Model file for the job. Use its own axes, mm. Round coordinates to 2 decimals unless told otherwise and drop trailing zeros. Order: outer loops, then holes, each group sorted by start corner. A loop starts at its lowest first (then second) coordinate and runs counter-clockwise, first axis right, second up. Notation, with made-up numbers: (22.25, 1) - (79.25, 1) arc R19 ccw to (79.25, 14) - close; hole circle Ø9 at (27.25, 5). An arc over 180 degrees is marked (long way). Write item = value, one per line. Start each with the question number.
from build123d import *

# Parameters (mm, degrees)
SKETCH1_W           = 51
SKETCH1_H           = 28
BOSS_EXTRUDE1_DEPTH = 3
SKETCH2_R           = 1.6
CUT_EXTRUDE1_DEPTH  = 3
SKETCH3_R           = 3.1
CUT_EXTRUDE2_DEPTH  = 3


with BuildPart() as part:
    # Sketch1 → Boss-Extrude1 (new body)
    with BuildSketch(Plane(origin=(0, 0, 0), x_dir=(1, 0, 0), z_dir=(0, 1, 0))):
        with Locations((-1.082278481, 0.240506329)):
            Rectangle(SKETCH1_W, SKETCH1_H)
    extrude(amount=BOSS_EXTRUDE1_DEPTH)

    # Sketch2 → Cut-Extrude1 (cut)
    with BuildSketch(Plane(origin=(0, 3, 0), x_dir=(1, 0, 0), z_dir=(0, 1, 0))):
        with Locations((-23.582278481, 11.240506329)):
            Circle(SKETCH2_R)
        with Locations((21.417721519, 11.240506329)):
            Circle(SKETCH2_R)
    extrude(amount=-CUT_EXTRUDE1_DEPTH, mode=Mode.SUBTRACT)

    # Sketch3 → Cut-Extrude2 (cut)
    with BuildSketch(Plane(origin=(0, 3, 0), x_dir=(1, 0, 0), z_dir=(0, 1, 0))):
        with Locations((-1.582278481, 0.240506329)):
            Circle(SKETCH3_R)
    extrude(amount=-CUT_EXTRUDE2_DEPTH, mode=Mode.SUBTRACT)


solid = part.part
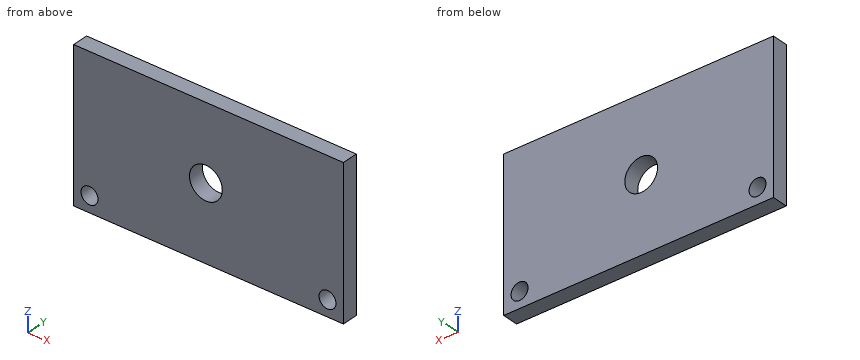
Item 1: Saw through at A-A, the plane z = -2.25. Give the cut face in (x, y).
Item 2: Drop flat-ended pins along their axis: pin 1 (8 mm diameter, centred on x = 4.5, z = 8, fed in from -Y); pin 2 (5.5 mm diameter, centred on x = -1.58, z = -0.24, fed in from -Y). Give the stop position or say it passes through.
Item 3: Probe L1, parallel to X at y = 2.4, z = -12.5; L2, parallel to X at y = 2.4, z = -10.5; L3, parallel to Z at x = 0.5, y = 1.65. List the from-to ranges inside material, lowest first.
Item 4: Saw through at B-B, the plane y = 0.9. Give the cut face in (x, z), then the cut area to 3 significant figures.
Item 5: Saw through at C-C, the plane x = -3.5. Give the cut face in (y, z), then the cut area to 3 significant figures.
Check sheet entries:
q1.outline = (-26.58, 0) - (-3.94, 0) - (-3.94, 3) - (-26.58, 3) - close; (0.78, 0) - (24.42, 0) - (24.42, 3) - (0.78, 3) - close
q2.pin_1 = 0
q2.pin_2 = through
q3.L1 = -26.58 to -24.57, -22.6 to 20.43, 22.4 to 24.42
q3.L2 = -26.58 to -25, -22.16 to 20, 22.84 to 24.42
q3.L3 = -14.24 to -2.54, 2.06 to 13.76
q4.outline = (-26.58, -14.24) - (24.42, -14.24) - (24.42, 13.76) - (-26.58, 13.76) - close; hole circle Ø3.2 at (-23.58, -11.24); hole circle Ø6.2 at (-1.58, -0.24); hole circle Ø3.2 at (21.42, -11.24)
q4.area = 1,380 mm2
q5.outline = (0, -14.24) - (3, -14.24) - (3, -2.68) - (0, -2.68) - close; (0, 2.2) - (3, 2.2) - (3, 13.76) - (0, 13.76) - close
q5.area = 69.4 mm2
